from build123d import *

# Parameters (mm, degrees)
F0_W        = 4.7625
F0_H        = 19.05
F1_DEPTH    = 12.7
F3_T1_DEPTH = 36.5125
F4_D        = 5.1054


# Not quite as in the source:
# - a fillet or chamfer that OpenCascade refuses, or shapes differently, is made with other operations: its cross-section is extruded or revolved along the edge and cut away or added


with BuildPart() as f1:
    # F0 (on Right) → F1 (new body)
    with BuildSketch(Plane.YZ):
        with Locations((2.38125, -9.525)):
            Rectangle(F0_W, F0_H)
    extrude(amount=F1_DEPTH)

    # F3: fillet of radius 6.35 on 2 edges, made by hand

    # F3_s2 → F3_t1 (cut)
    with BuildSketch(Plane.XZ.offset(-20.6375)):
        with BuildLine():
            add(Edge.make_bspline(
                [(6.35, 0), (0, 0), (0, -6.35)],
                knots=[0, 0, 0, 1, 1, 1], degree=2, weights=[1, 1, 1]))
            Line((0, -6.35), (0, 0))
            Line((0, 0), (6.35, 0))
        make_face()
        with BuildLine():
            add(Edge.make_bspline(
                [(6.35, 0), (12.7, 0), (12.7, -6.35)],
                knots=[0, 0, 0, 1, 1, 1], degree=2, weights=[1, 1, 1]))
            Line((12.7, -6.35), (12.7, 0))
            Line((12.7, 0), (6.35, 0))
        make_face()
    extrude(amount=F3_T1_DEPTH, mode=Mode.SUBTRACT)

    # F4 (through all)
    with Locations(Plane.XZ):
        with Locations((6.35, -6.35)):
            Hole(F4_D / 2)


solid = f1.part
Check sheet for the modelled part. Datum: model origin and axes. Units: mm. Round coordinates to 2 decimals unless told otherwise and drop trailing zeros. Loops run counter-clockwise (first coordinate to the right, second up) from the corner with the lowest first, then second, coordinate; pieces in that order, holes last.
1. Sectioned sample at A-A on z = -7.25. Record the boundary of the cut face in (x, y), and give its area (3 significant figures).
2. Scan lines: probe 1 along Z at (x, y) = (6.25, 2.85); probe 2 along Z at (x, y) = (7, 3.4); probe 3 along Z at (x, y) = (3, 3.6). Record each from-to range of solid material in increasing order.
3. Mould release check, pull along X, two halves, no side actions. Record for faces 1 (the cylindrical face through (4.978, 2.415, -4.198)), 2 (the flat face through (6, 2, -19.05)), 3 (the flat face through (0, 2, -13)): released by +X, released by -X, zero draft, split by the parting line, or undercut.
Recorded:
1. outline: (0, 0) - (3.96, 0) - (3.96, 4.76) - (0, 4.76) - close; (8.74, 0) - (12.7, 0) - (12.7, 4.76) - (8.74, 4.76) - close
1. area: 37.7 mm2
2. probe 1: z = -19.05 to -8.9, -3.8 to 0
2. probe 2: z = -19.05 to -8.82, -3.88 to -0.02
2. probe 3: z = -19.05 to -0.62
3. face 1: undercut
3. face 2: zero draft
3. face 3: released by -X
